Autodesk Inventor part; units mm, degrees
ref_plane "YZ Plane" through (0, 0, 0) normal (1, 0, 0) x (0, 1, 0)
ref_plane "XZ Plane" through (0, 0, 0) normal (0, 1, 0) x (-1, 0, 0)
ref_plane "XY Plane" through (0, 0, 0) normal (0, 0, 1) x (1, 0, 0)
sketch "Sketch1" plane through (0, 0, 0) normal (0, 1, 0) x (-1, 0, 0)
  circle A0 centre (0, 0) radius 28.6512 construction
  line L0 (0, 0) -> (0, 28.6512) construction
  line L1 (0, 0) -> (57.939, 0.3498) construction
  circle A1 centre (57.939, 0.3498) radius 9.5504 construction
  line L2 (61.0329, 9.3851) -> (9.2818, 27.1061)
  line L3 (61.1418, -8.6476) -> (9.6084, -26.992)
  arc A2 (61.1418, -8.6476) -> (61.0329, 9.3851) centre (57.939, 0.3498) ccw
  arc A3 (9.2818, 27.1061) -> (9.6084, -26.992) centre (0, 0) ccw
  line L4 (10.4602, -29.3849) -> (61.9936, -11.0405)
  arc A4 (61.9936, -11.0405) -> (61.8558, 11.7882) centre (57.939, 0.3498) ccw
  line L5 (61.8558, 11.7882) -> (10.1047, 29.5091)
  arc A5 (10.1047, 29.5091) -> (10.4602, -29.3849) centre (0, 0) ccw
  dimension "d0" = 57.3024
  dimension "d1" = 57.94
  dimension "d2" = 89.654
  dimension "d3" = 19.1008
  dimension "d4" = 2.54
extrude "Extrusion1" add sketch "Sketch1" along normal blind 8.9916
properties part number "INTK_009_Belt1" material "Rubber, Silicone"
Part model, mm, in its own coordinate system. A direction names the side the tool comes from. Round coordinates to 2 decimals unless told otherwise and drop trailing zeros. Write each loop counter-clockwise with the first axis right and the second up, starting at its lowest first coordinate (ties: lowest second). Pieces come first, ordered by that corner, then holes. Notation, with made-up numbers: M 43,28.5 L 87,28.5 A24 ccw 87,52.5 Z; hole C 68.5,79.5 d8. An arc over 180 degrees is marked long. Return JSON: item names as keys, results as strings. Group by question number.
(1) Saw through at A-A on z = -4. Write the cut outline in (x, y), then the cut area to 3 significant figures.
(2) Pin check, flat tips, straight feed: pin 1 Ø1.5 at (x, y) = (-43.5, 7) entering from -Z; pin 2 Ø1.5 at (y, z) = (4.5, -15.5) entering from +X; pin 3 Ø2 at (x, y) = (-42.5, 2) entering from +Z. Stop position of each tip, or through.
(3) Which spindle directions (+Z, -Z, +X, -X, +Y, -Y) get a long thin tool onto all of the face, cutting with end or side? Do faces 5 (the face through (-23, 8.992, -23)), 6 (the face through (-67.487, 4.433, 0.572)). Say none if no direction does.
(4) Saw through at B-B on y = 3.25. Write the cut outline in (x, z).
(5) Two-plate mould, pull along X, no slides. Class faces 1 (the face through (31.175, 4.433, -1.021)), 2 (the face through (-35.87, 4.43, -20.34)), 3 (the face through (-35.74, 4.43, -17.69)), 4 (the face through (-23, 0, -23)): +X half, -X half, draft (parallel to the pull), parting line (faces both ways), or undercut.
(6) Drill centre lines: probe 1 along Z at (x, y) = (-27, 2.25); probe 2 along Z at (x, y) = (-66, 7.5); probe 3 along X at (y, z) = (2, 4.5). Where is each one in solid material? Low to high.
(7) Saw through at C-C on x = -48. Write the cut outline in (y, z), then the cut area to 3 significant figures.
Returned:
{
 "1": {"outline": "M -69.22,0 L -66.44,0 L -66.44,8.99 L -69.22,8.99 Z; M 28.37,0 L 30.93,0 L 30.93,8.99 L 28.37,8.99 Z", "area": "48.0 mm²"},
 "2": {"pin 1": "z = -17.89", "pin 2": "x = 27.48", "pin 3": "z = 18.76"},
 "3": {"face 5": "+Z, -Z, +X, -X, +Y", "face 6": "+Y, -Y"},
 "4": {"outline": "M -61.99,-11.04 L -10.46,-29.38 A31.19 ccw long -10.1,29.51 L -61.86,11.79 A12.09 ccw Z; hole M -61.14,-8.65 L -9.61,-26.99 A28.65 ccw long -9.28,27.11 L -61.03,9.39 A9.55 ccw Z"},
 "5": {"face 1": "parting line", "face 2": "-X half", "face 3": "undercut", "face 4": "draft"},
 "6": {"probe 1": "-23.5 to -20.8, 21.04 to 23.72", "probe 2": "-8.66 to -4.77, 5.47 to 9.36", "probe 3": "-69.29 to -66.54, 28.3 to 30.86"},
 "7": {"outline": "M 0,-16.02 L 8.99,-16.02 L 8.99,-13.33 L 0,-13.33 Z; M 0,13.85 L 8.99,13.85 L 8.99,16.53 L 0,16.53 Z", "area": "48.4 mm²"}
}
